Here's how the part is built. I have some questions about the finished solid (model axes, mm). Face numbers are marked on the shaded views. A direction names the side the tool comes from. Give positions to 0.01 mm unless a question says otherwise; leave off trailing zeros. Loops run counter-clockwise (first coordinate to the right, second up) from the corner with the lowest first, then second, coordinate; pieces in that order, holes last. Notation, with made-up numbers: (38, -29.75) - (48, -29.75) arc R34 ccw to (48, 6.25) - close; hole circle Ø4 at (28, 47.25). An arc over 180 degrees is marked (long way). Use one line per item in the form item = value.
Autodesk Inventor part; units mm, degrees
ref_plane "YZ Plane" through (0, 0, 0) normal (1, 0, 0) x (0, 1, 0)
ref_plane "XZ Plane" through (0, 0, 0) normal (0, 1, 0) x (-1, 0, 0)
ref_plane "XY Plane" through (0, 0, 0) normal (0, 0, 1) x (1, 0, 0)
sketch "Boceto1" plane through (0, 0, 0) normal (0, 1, 0) x (-1, 0, 0)
  line L0 (0, 0) -> (-10, 0)
  line L1 (-10, -20) -> (0, -20)
  line L2 (-10, 0) -> (-8, 0)
  line L3 (-8, 0) -> (-14, 0)
  line L4 (-14, 0) -> (-18, 0)
  line L5 (-18, 0) -> (-18, -20)
  line L6 (-18, -20) -> (-10, -20)
  line L7 (0, -20) -> (-2, -20)
  line L8 (-2, -20) -> (6, -20)
  line L9 (6, -20) -> (6, 0)
  line L10 (6, 0) -> (0, 0)
  dimension "d8" = 4
  dimension "d9" = 8
extrude "Extrusión1" add sketch "Boceto1" along normal blind 3
sketch "Boceto2" plane through (0, 3, 0) normal (0, 1, 0) x (1, 0, 0)
  line L0 (5, 20) -> (2, 20)
  line L1 (2, 0) -> (2, 20)
  line L2 (5, 20) -> (8, 20)
  line L3 (8, 0) -> (8, 20)
  line L4 (2, 0) -> (8, 0)
extrude "Extrusión2" add sketch "Boceto2" along normal blind 50
sketch "Boceto4" plane through (0, 3, 0) normal (0, 1, 0) x (1, 0, 0)
  line L0 (-6, 0) -> (18, 0)
  line L1 (18, 0) -> (8, 0)
  line L2 (13, 0) -> (13, 20)
  point P0 (0, 0)
  point P1 (13, 10)
hole "Agujero2" at (13, 3, -10) direction (0, -1, 0) diameter 3.2 depth 15 counterbore diameter 6 counterbore depth 2
sketch "Boceto5" plane through (0, 3, 0) normal (0, 1, 0) x (1, 0, 0)
  line L0 (-6, 20) -> (-6, 0)
  line L1 (-6, 10) -> (2, 10)
  point P0 (0, 0)
  point P1 (-2, 10)
hole "Agujero3" at (-2, 3, -10) direction (0, -1, 0) diameter 3.2 depth 15 counterbore diameter 6 counterbore depth 2
sketch "Boceto6" plane through (8, 3, 0) normal (1, 0, 0) x (0, 0, -1)
  line L0 (10, 10) -> (11.6, 10)
  line L1 (10, 10) -> (8.4, 10)
  line L2 (8.4, 10) -> (8.4, 40)
  line L3 (11.6, 40) -> (11.6, 10)
  line L4 (11.6, 40) -> (11.6, 45)
  line L5 (11.6, 45) -> (8.4, 45)
  line L6 (8.4, 45) -> (8.4, 40)
  point P0 (0, -3)
extrude "Extrusión3" cut sketch "Boceto6" against normal blind 35.5
fillet "Empalme1" radius 1.6 4 edges at (5, 48, -11.6) (5, 48, -8.4) (5, 13, -8.4) (5, 13, -11.6)
properties part number "Ventilador tub - guies"
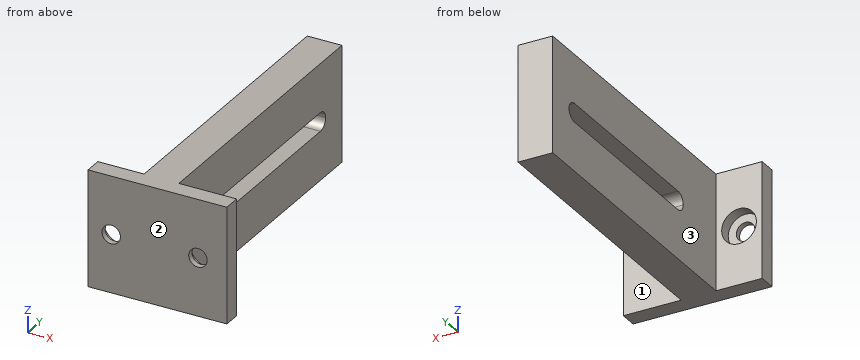
(1) If we section it at C-C (z = -10.5): List the corners of the cut face in (x, y) for me.
Geometry says:
outline = (-6, 0) - (-3.52, 0) - (-3.52, 1) - (-4.96, 1) - (-4.96, 3) - (-6, 3) - close; (-0.48, 0) - (11.48, 0) - (11.48, 1) - (10.04, 1) - (10.04, 3) - (8, 3) - (8, 13.08) - (2, 13.08) - (2, 3) - (0.96, 3) - (0.96, 1) - (-0.48, 1) - close; (2, 47.92) - (8, 47.92) - (8, 53) - (2, 53) - close; (14.52, 0) - (18, 0) - (18, 3) - (15.96, 3) - (15.96, 1) - (14.52, 1) - close
(2) If we section it at A-A (y = 44): List the corners of the cut face in (x, z) for me.
Geometry says:
outline = (2, -20) - (8, -20) - (8, -11.6) - (2, -11.6) - close; (2, -8.4) - (8, -8.4) - (8, 0) - (2, 0) - close
(3) If I drill on probe 1 along X at (y, z) = (2.4, -10); probe 2 along X at (y, z) = (0.7, -10); probe 3 along Z at (x, y) = (6.5, 26), over which ranges is the centre line in solid material (lowest first)?
Geometry says:
probe_1 = -6 to -5, 1 to 10, 16 to 18
probe_2 = -6 to -3.6, -0.4 to 11.4, 14.6 to 18
probe_3 = -20 to -11.6, -8.4 to 0
(4) For the marked faces 1, 2 and 3, which set-ups out of +Z, -Z, +X, -X, +Y, -Y let a thin tool reach every point of the face, with its end or its side?
Geometry says:
face_1 = +Z, -Z, +X, +Y
face_2 = +Z, -Z, +X, -X, -Y
face_3 = +Z, -Z, -X, +Y
(5) If we section it at B-B (x = 13): List the corners of the cut face in (y, z) for me.
Geometry says:
outline = (0, -20) - (3, -20) - (3, -13) - (1, -13) - (1, -11.6) - (0, -11.6) - close; (0, -8.4) - (1, -8.4) - (1, -7) - (3, -7) - (3, 0) - (0, 0) - close
(6) For P1, Ø6.5, axis at x = 13, z = -9, coming from the +Y side; P2, Ø10, axis at y = 25, z = -13.5, coming from the +X side; P3, Ø3, axis at x = -3, z = -9, coming from the +Y side, each with a flat end and sliding along its axis, tell me the tip position at first contact or that it passes through.
Geometry says:
P1 = 3
P2 = 8
P3 = 1
